```python
from build123d import *

# Parameters (mm, degrees)
SKETCH_4_R          = 1.4
SKETCH_4_R_2        = 1.65
EXTRUDE_1_DEPTH     = 3
SKETCH_5_W          = 12.6
SKETCH_5_H          = 12.6
EXTRUDE_2_DEPTH     = 30
SKETCH_6_W          = 9
SKETCH_6_H          = 8
SKETCH_6_W_2        = 8
SKETCH_6_H_2        = 9
CUT_EXTRUDE_2_DEPTH = 71.809603868
EXTRUDE_3_DEPTH     = 3
EXTRUDE_4_DEPTH     = 3
EXTRUDE_5_DEPTH     = 3
EXTRUDE_6_DEPTH     = 3
SKETCH_13_W         = 12.6
SKETCH_13_H         = 12.6
EXTRUDE_7_DEPTH     = 22
SKETCH_14_R         = 1.4
SKETCH_14_R_2       = 1.65
EXTRUDE_8_DEPTH     = 3
SKETCH_15_W         = 13.5
SKETCH_15_H         = 10
CUT_EXTRUDE_3_DEPTH = 84.366660003


with BuildPart() as part:
    # 草图4 → 凸台-拉伸1 (new body)
    with BuildSketch(Plane.XY):
        Polygon((-39, 30), (20, 30), (20, 19), (5, 19), (5, -19), (20, -19), (20, -30), (-39, -30), (-55, -30), (-55, 30), align=None)
        with Locations((-49.5, 24.5)):
            Circle(SKETCH_4_R, mode=Mode.SUBTRACT)
        with Locations((8.5, 24.5)):
            Circle(SKETCH_4_R, mode=Mode.SUBTRACT)
        with Locations((-3, 26)):
            Circle(SKETCH_4_R_2, mode=Mode.SUBTRACT)
        with Locations((-37, 26)):
            Circle(SKETCH_4_R_2, mode=Mode.SUBTRACT)
        with Locations(Location((-37, -26, 0), (0, 0, 180))):
            Circle(SKETCH_4_R_2, mode=Mode.SUBTRACT)
        with Locations(Location((-3, -26, 0), (0, 0, 180))):
            Circle(SKETCH_4_R_2, mode=Mode.SUBTRACT)
        with Locations(Location((8.5, -24.5, 0), (0, 0, 180))):
            Circle(SKETCH_4_R, mode=Mode.SUBTRACT)
        with Locations(Location((-49.5, -24.5, 0), (0, 0, 180))):
            Circle(SKETCH_4_R, mode=Mode.SUBTRACT)
    extrude(amount=EXTRUDE_1_DEPTH)

    # 草图5 → 凸台-拉伸2 (add)
    with BuildSketch(Plane.XY.offset(3)):
        with Locations((-17.5, 0)):
            Rectangle(SKETCH_5_W, SKETCH_5_H)
    extrude(amount=EXTRUDE_2_DEPTH)

    # 草图6 → 切除-拉伸2 (cut, through all)
    with BuildSketch(Plane(origin=(0, 0, 0), x_dir=(-1, 0, 0), z_dir=(0, 0, -1))):
        with Locations((17.5, 13)):
            Rectangle(SKETCH_6_W, SKETCH_6_H)
        with Locations((30.5, 0)):
            Rectangle(SKETCH_6_W_2, SKETCH_6_H_2)
        with Locations((17.5, -13)):
            Rectangle(SKETCH_6_W, SKETCH_6_H)
        with Locations((4.5, 0)):
            Rectangle(SKETCH_6_W_2, SKETCH_6_H_2)
    extrude(amount=-CUT_EXTRUDE_2_DEPTH, mode=Mode.SUBTRACT)

    # 草图8 → 凸台-拉伸3 (add)
    with BuildSketch(Plane(origin=(-11.2, 0, 0), x_dir=(0, 0, -1), z_dir=(1, 0, 0))):
        Polygon((-31, 4.3), (-22.4, 4.3), (-22.4, 6.3), (-33, 6.3), (-33, -6.3), (-22.4, -6.3), (-22.4, -4.3), (-31, -4.3), align=None)
    extrude(amount=EXTRUDE_3_DEPTH)

    # 草图10 → 凸台-拉伸4 (add)
    with BuildSketch(Plane.ZY.offset(23.8)):
        Polygon((22.4, 6.3), (22.4, 4.3), (31, 4.3), (31, -4.3), (22.4, -4.3), (22.4, -6.3), (33, -6.3), (33, 6.3), align=None)
    extrude(amount=EXTRUDE_4_DEPTH)

    # 草图11 → 凸台-拉伸5 (add)
    with BuildSketch(Plane.XZ.offset(6.3)):
        Polygon((-23.8, 22.4), (-23.8, 33), (-11.2, 33), (-11.2, 22.4), (-13.2, 22.4), (-13.2, 31), (-21.8, 31), (-21.8, 22.4), align=None)
    extrude(amount=EXTRUDE_5_DEPTH)

    # 草图12 → 凸台-拉伸6 (add)
    with BuildSketch(Plane(origin=(0, 6.3, 0), x_dir=(1, 0, 0), z_dir=(0, 1, 0))):
        Polygon((-23.8, -22.4), (-23.8, -33), (-11.2, -33), (-11.2, -22.4), (-13.2, -22.4), (-13.2, -31), (-21.8, -31), (-21.8, -22.4), align=None)
    extrude(amount=EXTRUDE_6_DEPTH)

    # 草图13 → 凸台-拉伸7 (add)
    with BuildSketch(Plane.XY.offset(33)):
        with Locations((-17.5, 0)):
            Rectangle(SKETCH_13_W, SKETCH_13_H)
    extrude(amount=EXTRUDE_7_DEPTH)

    # 草图14 → 凸台-拉伸8 (add)
    with BuildSketch(Plane.XY.offset(55)):
        Polygon((-39, 30), (20, 30), (20, -30), (-39, -30), (-55, -30), (-55, 30), align=None)
        with Locations((-49.5, 24.5)):
            Circle(SKETCH_14_R, mode=Mode.SUBTRACT)
        with Locations((8.5, 24.5)):
            Circle(SKETCH_14_R, mode=Mode.SUBTRACT)
        with Locations((-3, 26)):
            Circle(SKETCH_14_R_2, mode=Mode.SUBTRACT)
        with Locations((-37, 26)):
            Circle(SKETCH_14_R_2, mode=Mode.SUBTRACT)
        with Locations(Location((-37, -26, 0), (0, 0, 180))):
            Circle(SKETCH_14_R_2, mode=Mode.SUBTRACT)
        with Locations(Location((-3, -26, 0), (0, 0, 180))):
            Circle(SKETCH_14_R_2, mode=Mode.SUBTRACT)
        with Locations(Location((8.5, -24.5, 0), (0, 0, 180))):
            Circle(SKETCH_14_R, mode=Mode.SUBTRACT)
        with Locations(Location((-49.5, -24.5, 0), (0, 0, 180))):
            Circle(SKETCH_14_R, mode=Mode.SUBTRACT)
    extrude(amount=EXTRUDE_8_DEPTH)

    # 草图15 → 切除-拉伸3 (cut, through all)
    with BuildSketch(Plane.XY.offset(3)):
        with Locations((-1.75, 14)):
            Rectangle(SKETCH_15_W, SKETCH_15_H)
        with Locations((-1.75, -14)):
            Rectangle(SKETCH_15_W, SKETCH_15_H)
    extrude(amount=-CUT_EXTRUDE_3_DEPTH, mode=Mode.SUBTRACT)


solid = part.part
```
CAD build for the part. Positions are in the model's coordinates, mm. A direction names the side the tool comes from. Round coordinates to 2 decimals unless told otherwise and drop trailing zeros. Order: outer loops, then holes, each group sorted by start corner. A loop starts at its lowest first (then second) coordinate and runs counter-clockwise, first axis right, second up. Notation, with made-up numbers: (73, 78) -> (119, 78) arc R12 ccw to (119, 95) -> close; hole circle Ø9 at (33.5, 67). An arc over 180 degrees is marked (long way). One line per question, with ' | ' between items.
Q1. Drop flat-ended pins along their axis: pin 1 (10 mm diameter, centred on y = 8.5, z = 33.5, fed in from +X); pin 2 (2 mm diameter, centred on x = -37, y = 26, fed in from -Z); pin 3 (2.5 mm diameter, centred on y = 16.5, z = 2, fed in from +X); pin 4 (14 mm diameter, centred on x = -18.5, z = 44.5, fed in from -Y). Give the stop position or say it passes through.
Completed:
pin 1: stops at x = -8.2 | pin 2: passes through | pin 3: stops at x = -8.5 | pin 4: stops at y = -6.3
Q2. Slice it at D-D (y = 12). Write the cut outline in (x, z), then the cut area to 4 significant figures.
Completed:
outline: (-55, 0) -> (-22, 0) -> (-22, 3) -> (-55, 3) -> close; (-55, 55) -> (20, 55) -> (20, 58) -> (-55, 58) -> close; (-13, 0) -> (-8.5, 0) -> (-8.5, 3) -> (-13, 3) -> close | area: 337.5 mm^2
Q3. Slice it at A-A (x = -29.5). Write the cut outline in (y, z).
Completed:
outline: (-30, 0) -> (-4.5, 0) -> (-4.5, 3) -> (-30, 3) -> close; (-30, 55) -> (30, 55) -> (30, 58) -> (-30, 58) -> close; (4.5, 0) -> (30, 0) -> (30, 3) -> (4.5, 3) -> close
Q4. Probe probe 1 along Y at (x, z) = (-3, 57); probe 2 along Y at (x, z) = (-49.5, 55.75); probe 3 along Z at (x, y) = (-21, 17.5). List the from-to ranges inside material, lowest first.
Completed:
probe 1: y = -30 to -27.65, -24.35 to 24.35, 27.65 to 30 | probe 2: y = -30 to -25.9, -23.1 to 23.1, 25.9 to 30 | probe 3: z = 0 to 3, 55 to 58
Q5. Slice it at B-B (x = -49.5). Write the cut outline in (y, z), then the cut area to 3 significant figures.
Completed:
outline: (-30, 0) -> (-25.9, 0) -> (-25.9, 3) -> (-30, 3) -> close; (-30, 55) -> (-25.9, 55) -> (-25.9, 58) -> (-30, 58) -> close; (-23.1, 0) -> (23.1, 0) -> (23.1, 3) -> (-23.1, 3) -> close; (-23.1, 55) -> (23.1, 55) -> (23.1, 58) -> (-23.1, 58) -> close; (25.9, 0) -> (30, 0) -> (30, 3) -> (25.9, 3) -> close; (25.9, 55) -> (30, 55) -> (30, 58) -> (25.9, 58) -> close | area: 326 mm^2
Q6. Slice it at C-C (y = -18). Write the cut outline in (x, z), then the cut area to 4 significant figures.
Completed:
outline: (-55, 0) -> (-8.5, 0) -> (-8.5, 3) -> (-55, 3) -> close; (-55, 55) -> (20, 55) -> (20, 58) -> (-55, 58) -> close | area: 364.5 mm^2
Q7. Which spindle directions (+Z, -Z, +X, -X, +Y, -Y) get a long thin tool onto all of the face, cutting with end or side? Do faces 4 (the flat face through (-17.6, 9.3, 31.2)), 5 (the flat face through (-23, -8, 22.4)), 6 (the flat face through (-8.5, 14, 2)), 7 (the flat face through (-10, -4.3, 27)), 8 (the flat face through (-30, -4.5, 1)). Say none if no direction does.
Completed:
face 4: +X, -X, +Y | face 5: +X, -X, -Y | face 6: -Z, +X | face 7: +X | face 8: -Z
Q8. Two-plate mould, pull along Y, no slides. Class faces 1 (the flat face through (-17, 30, 1)), 2 (the flat face through (-10, -5, 22.4)), 3 (the flat face through (-25, 4.3, 27)): released by +Y, released by -Y, zero draft, split by the parting line, or undercut.
Completed:
face 1: released by +Y | face 2: zero draft | face 3: undercut
